Geometry: see drawing. Coordinates: mm, zero at the bounding-box minimum. A direction names the side the tool comes from. Coordinates: 2 decimals unless noted, no trailing zeros. Loops run counter-clockwise (first coordinate to the right, second up) from the corner with the lowest first, then second, coordinate; pieces in that order, holes last. Notation, with made-up numbers: (25.25, -19.75) -> (67.25, -19.75) arc R21 cw to (67.25, 16.25) -> close; hole circle Ø5 at (-23, 2). An arc over 180 degrees is marked (long way). Put each result on its own line as item: value. Start each with the question number.
1) Cut plane D-D (z = 1.25). Return the cut outline in (x, y), plus the area to 3 significant figures.
2) Contact query for flat-ended pins moving along their axis: P1, Ø3.5, axis at x = 3.5, z = 5.5, coming from the -Y side; P2, Ø0.6, axis at y = 15.5, z = 1, coming from the +X side; P3, Ø6, axis at x = 5, y = 9.5, coming from the -Z side; P4, Ø10, axis at x = 10.5, y = 16, coming from the -Z side. Output: stop coordinate, or through.
3) Cut plane B-B (x = 3). Return the cut outline in (y, z), plus the area to 3 significant figures.
4) Material intervals for L1, parallel to Z at x = 14.5, y = 13.25; L2, parallel to Z at x = 6, y = 10.25; L3, parallel to Y at x = 13.5, z = 3.5, sorted ascending.
5) Cut plane C-C (z = 3.5). Return the cut outline in (x, y), plus the area to 3 significant figures.
6) Set-up query: the marked faces 1, 2, 3 and 4. Return all of +Z, -Z, +X, -X, +Y, -Y with unobstructed straight access to the full face (end or side cutting, diameter ignored); none if empty.
7) Cut plane A-A (y = 14.5). Return the cut outline in (x, z), plus the area to 3 significant figures.
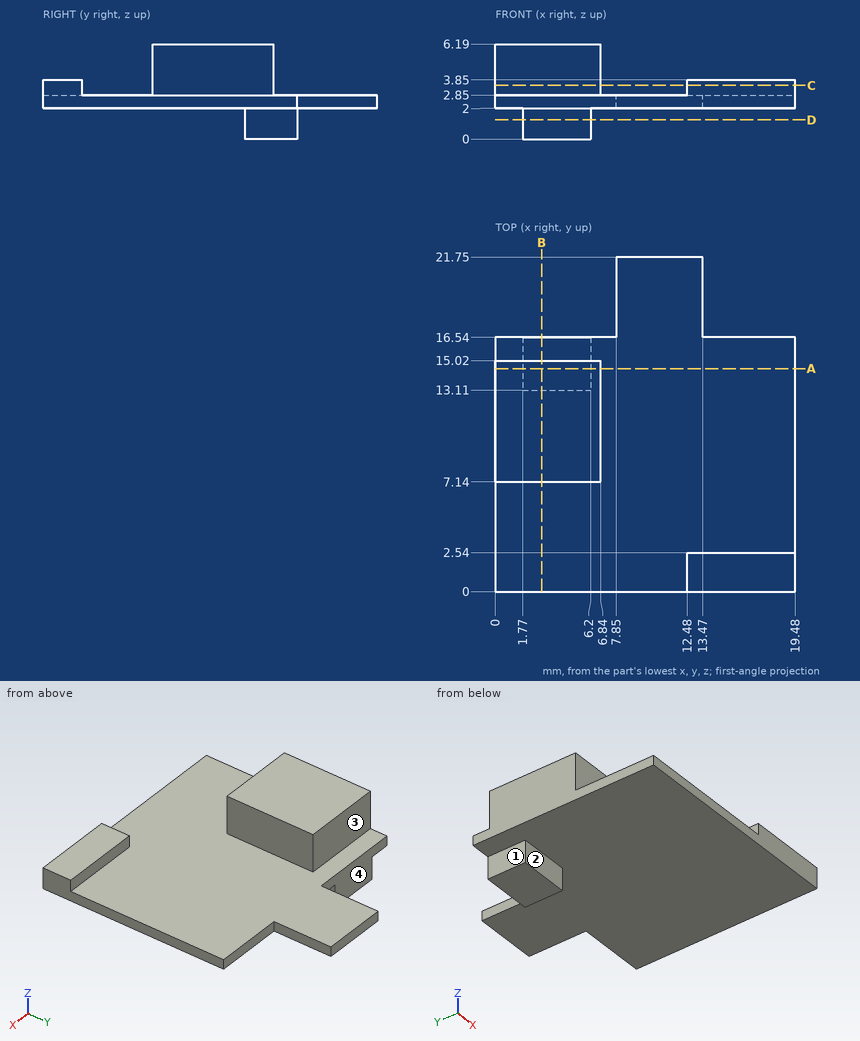
Results found:
1. outline: (1.77, 13.11) -> (6.2, 13.11) -> (6.2, 16.54) -> (1.77, 16.54) -> close
1. area: 15.2 mm2
2. P1: stops at y = 7.14
2. P2: stops at x = 6.2
2. P3: stops at z = 2
2. P4: stops at z = 0
3. outline: (0, 2) -> (13.11, 2) -> (13.11, 0) -> (16.54, 0) -> (16.54, 2.85) -> (15.02, 2.85) -> (15.02, 6.19) -> (7.14, 6.19) -> (7.14, 2.85) -> (0, 2.85) -> close
3. area: 47.2 mm2
4. L1: z = 2 to 2.85
4. L2: z = 2 to 6.19
4. L3: y = 0 to 2.54
5. outline: (0, 7.14) -> (6.84, 7.14) -> (6.84, 15.02) -> (0, 15.02) -> close; (12.48, 0) -> (19.48, 0) -> (19.48, 2.54) -> (12.48, 2.54) -> close
5. area: 71.7 mm2
6. face 1: -Z, -X, +Y, -Y
6. face 2: -Z, +X, -X, -Y
6. face 3: +Z, +X, -X, +Y
6. face 4: +Z, -Z, -X, +Y
7. outline: (0, 2) -> (1.77, 2) -> (1.77, 0) -> (6.2, 0) -> (6.2, 2) -> (19.48, 2) -> (19.48, 2.85) -> (6.84, 2.85) -> (6.84, 6.19) -> (0, 6.19) -> close
7. area: 48.3 mm2
